```python
from build123d import *

# Parameters (mm, degrees)
SKETCH1_W           = 79.375
SKETCH1_H           = 66.675
SKETCH1_W_2         = 73.025
SKETCH1_H_2         = 60.325
EXTRUDE_THIN1_DEPTH = 73.025
FILLET1_R           = 9.525
BOSS_EXTRUDE1_DEPTH = 3.175
FILLET2_R           = 6.35
FILLET3_R           = 1.5875


with BuildPart() as part:
    # Sketch1 → Extrude-Thin1 (new body)
    with BuildSketch(Plane(origin=(0, 0, 0), x_dir=(1, 0, 0), z_dir=(0, 1, 0))):
        Rectangle(SKETCH1_W, SKETCH1_H)
        Rectangle(SKETCH1_W_2, SKETCH1_H_2, mode=Mode.SUBTRACT)
    extrude(amount=EXTRUDE_THIN1_DEPTH)

    # Fillet1
    fillet1_edges = [part.edges().sort_by_distance(p)[0] for p in [
        (36.5125, 36.5125, 30.1625),
        (36.5125, 36.5125, -30.1625),
        (-36.5125, 36.5125, -30.1625),
        (-36.5125, 36.5125, 30.1625),
        (39.6875, 36.5125, 33.3375),
        (-39.6875, 36.5125, 33.3375),
        (-39.6875, 36.5125, -33.3375),
        (39.6875, 36.5125, -33.3375),
    ]]
    fillet(fillet1_edges, radius=FILLET1_R)

    # Sketch2 → Boss-Extrude1 (add)
    with BuildSketch(Plane.XZ):
        with BuildLine():
            Line((39.6875, -23.8125), (39.6875, 23.8125))
            ThreePointArc((39.6875, 23.8125), (36.897692091, 30.547692091), (30.1625, 33.3375))
            Line((30.1625, 33.3375), (-30.1625, 33.3375))
            ThreePointArc((-30.1625, 33.3375), (-36.897692091, 30.547692091), (-39.6875, 23.8125))
            Line((-39.6875, 23.8125), (-39.6875, -23.8125))
            ThreePointArc((-39.6875, -23.8125), (-36.897692091, -30.547692091), (-30.1625, -33.3375))
            Line((-30.1625, -33.3375), (30.1625, -33.3375))
            ThreePointArc((30.1625, -33.3375), (36.897692091, -30.547692091), (39.6875, -23.8125))
        make_face()
    extrude(amount=BOSS_EXTRUDE1_DEPTH)

    # Fillet2
    fillet2_edges = [part.edges().sort_by_distance(p)[0] for p in [
        (-36.5125, 0, 0),
        (0, 0, 30.1625),
        (36.5125, 0, 0),
        (0, 0, -30.1625),
        (-33.722692091, 0, 27.372692091),
        (33.722692091, 0, 27.372692091),
        (33.722692091, 0, -27.372692091),
        (-33.722692091, 0, -27.372692091),
    ]]
    fillet(fillet2_edges, radius=FILLET2_R)

    # Fillet3
    fillet3_edges = [part.edges().sort_by_distance(p)[0] for p in [
        (-36.5125, 73.025, 0),
        (0, 73.025, 30.1625),
        (36.5125, 73.025, 0),
        (0, 73.025, -30.1625),
        (39.6875, 73.025, 0),
        (0, 73.025, 33.3375),
        (0, 73.025, -33.3375),
        (-39.6875, 73.025, 0),
        (36.897692091, 73.025, -30.547692091),
        (-36.897692091, 73.025, -30.547692091),
        (-36.897692091, 73.025, 30.547692091),
        (36.897692091, 73.025, 30.547692091),
        (-33.722692091, 73.025, 27.372692091),
        (33.722692091, 73.025, 27.372692091),
        (33.722692091, 73.025, -27.372692091),
        (-33.722692091, 73.025, -27.372692091),
        (36.897692091, -3.175, -30.547692091),
        (39.6875, -3.175, 0),
        (36.897692091, -3.175, 30.547692091),
        (0, -3.175, 33.3375),
        (-36.897692091, -3.175, 30.547692091),
        (-39.6875, -3.175, 0),
        (-36.897692091, -3.175, -30.547692091),
        (0, -3.175, -33.3375),
    ]]
    fillet(fillet3_edges, radius=FILLET3_R - 0.0001)  # a hair under: the kernel refuses the full size

    # Sketch4 → Cut-Revolve1 (revolve, cut)
    with BuildSketch(Plane.YX.offset(19.05), mode=Mode.PRIVATE) as cut_revolve1_sk:
        Polygon((-3.175, -23.33625), (-1.240026103, -23.33625), (0, -21.2725), (0, -25.4), (-3.175, -25.4), align=None)
    cut_revolve1 = revolve(cut_revolve1_sk.sketch.rotate(Axis((-25.4, 0, -19.05), (0, -1, 0)), 90), axis=Axis((-25.4, 0, -19.05), (0, -1, 0)), mode=Mode.SUBTRACT)

    # Mirror1: Cut-Revolve1 across plane
    add(cut_revolve1.mirror(Plane(origin=(0, 0, 0), x_dir=(0, 0, 1), z_dir=(1, 0, 0))), mode=Mode.SUBTRACT)

    # Mirror2: Cut-Revolve1 across plane
    add(cut_revolve1.mirror(Plane.XY), mode=Mode.SUBTRACT)

    # Mirror2 copy 1 sketch → Mirror2 copy 1 (revolve, cut)
    with BuildSketch(Plane(origin=(0, 0, 19.05), x_dir=(0, 1, 0), z_dir=(0, 0, 1))):
        Polygon((-3.175, -23.33625), (-1.240026103, -23.33625), (0, -21.2725), (0, -25.4), (-3.175, -25.4), align=None)
    revolve(axis=Axis((25.4, 0, 19.05), (0, -1, 0)), mode=Mode.SUBTRACT)


solid = part.part
```
Here's how the part is built. I have some questions about the finished solid (model axes, mm). A direction names the side the tool comes from. Coordinates: 2 decimals unless noted, no trailing zeros. One line per question, with ' | ' between items. Start each with the question number.
1. If we section it at A-A (z = -19.05): Give the number of separate pieces and of enclosed holes in the cut face, and give its area (3 significant figures).
2. I'm going to push flat-ended pins straight in: pin 1 Ø2 at (x, z) = (24.5, -20.5) entering from +Y; pin 2 Ø3.5 at (x, z) = (25.4, -19.05) entering from +Y; pin 3 Ø24 at (x, z) = (13.5, 11.5) entering from +Y; pin 4 Ø4.5 at (x, z) = (-25.4, 19.05) entering from -Y (3 decimals). Where does each tip first touch, or does it pass through?
3. Please list where these lines run through material, in increasing order: line 1 along Z through (x, y) = (-10, 46); line 2 along X through (y, z) = (11.5, -11); line 3 along X through (y, z) = (-2, -19). Write a range as [from, to].
4. Which directions (+Z, -Z, +X, -X, +Y, -Y) give clear straight access to the entire face, cutting with the end or side of a thin tool? Please do faces 1 (the flat face through (0, 35, -33.338)), 2 (the cylindrical face through (-34.7, 1.91, -0.29)).
5. If we mould it in two halves opening along X, with no side actions, what happens to faces 3 (the conical face through (26.88, -1.16, -20.67)), 4 (the flat face through (0, 35, 33.338)), 5 (the flat face through (39.688, 35, 0))? For each: released by +X, released by -X, zero draft, split by the parting line, or undercut.
Model answer:
1) separate pieces: 3 | enclosed holes: 0 | area: 698 mm²
2) pin 1: stops at y = -0.85 | pin 2: passes through | pin 3: stops at y = 0 | pin 4: stops at y = -3.175
3) line 1: z = [-33.34, -30.16], [30.16, 33.34] | line 2: x = [-39.69, -36.51], [36.51, 39.69] | line 3: x = [-39.63, -27.46], [-23.34, 23.34], [27.46, 39.63]
4) face 1: -Z, +X, -X, +Y, -Y | face 2: +Y
5) face 3: undercut | face 4: zero draft | face 5: released by +X
